Geometry check sheet. Reference: the model listing, model coordinates, mm. Face numbers are marked on the shaded views. A direction names the side the tool comes from. Give positions to 0.01 mm unless a question says otherwise; leave off trailing zeros. Write each loop counter-clockwise with the first axis right and the second up, starting at its lowest first coordinate (ties: lowest second). Pieces come first, ordered by that corner, then holes.
(1) Depth check by flat-ended pin: P1, Ø1.8, axis at x = 0, y = 6, coming from the -Z side; P2, Ø10, axis at x = 8, z = 18, coming from the +Y side; P3, Ø10, axis at x = 9.5, z = 1.5, coming from the +Y side; P4, Ø1.5, axis at x = 3, z = 2.5, coming from the +Y side. Enter the tip coordinate at first touch or a pass-through.
(2) Mould release check, pull along X, two halves, no side actions. Record for the marked faces 1, 2 and 3: +X half, -X half, draft (parallel to the pull), parting line (faces both ways), or undercut.
(3) Cross-section at A-A (y = 0). Record the boundary of the cut face in (x, z), and give its area (3 significant figures).
(4) Cross-section at D-D (x = -13). Record the boundary of the cut face in (y, z).
(5) Cross-section at C-C (x = -6.5). Record the boundary of the cut face in (y, z).
(6) Cross-section at B-B (x = 0). Record the boundary of the cut face in (y, z).
(7) Thickness scan on line 1 along Y through (x, z) = (0, 11); line 2 along Z through (x, y) = (3, 6); line 3 along X through (y, z) = (5, 3.5). Record the ranges inside material, lowest first.
(8) Tool access check on the marked faces 4, 5, 6, 7 and 8. Record the directions out of +Z, -Z, +X, -X, +Y, -Y that give a thin tool (end or side, any length) a straight path to the whole face; none if there is none.
```python
from build123d import *

# Parameters (mm, degrees)
SKIZZE1_R                       = 6
AUFSATZ_LINEAR_AUSTRAGEN1_DEPTH = 9
SKIZZE2_R                       = 3.925
AUFSATZ_LINEAR_AUSTRAGEN2_DEPTH = 7
SKIZZE3_R                       = 21
AUFSATZ_LINEAR_AUSTRAGEN3_DEPTH = 19
SKIZZE4_R                       = 15
SCHNITT_LINEAR_AUSTRAGEN2_DEPTH = 15.2
AUFSATZ_LINEAR_START            = -19
AUFSATZ_LINEAR_AUSTRAGEN4_DEPTH = 19
KREISMUSTER1_COUNT              = 9
SKETCH1_R                       = 1.5
CUT_EXTRUDE1_DEPTH              = 41.448579025
CUT_EXTRUDE2_START              = -3.8
SKETCH2_R                       = 2.25
CUT_EXTRUDE2_DEPTH              = 37.648579025
CUT_EXTRUDE3_START              = -3.8
CUT_EXTRUDE3_DEPTH              = 3.8


# Read off the part's stored shape, not the designer's step: Cut-Extrude3
with BuildPart() as part:
    # Skizze1 → Aufsatz-Linear austragen1 (new body)
    with BuildSketch(Plane.XY):
        Circle(SKIZZE1_R)
    extrude(amount=AUFSATZ_LINEAR_AUSTRAGEN1_DEPTH)

    # Skizze2 → Aufsatz-Linear austragen2 (add)
    with BuildSketch(Plane(origin=(0, 0, 0), x_dir=(-1, 0, 0), z_dir=(0, 0, -1))):
        Circle(SKIZZE2_R)
    extrude(amount=AUFSATZ_LINEAR_AUSTRAGEN2_DEPTH)

    # Skizze3 → Aufsatz-Linear austragen3 (add)
    with BuildSketch(Plane.XY.offset(9)):
        Circle(SKIZZE3_R)
    extrude(amount=AUFSATZ_LINEAR_AUSTRAGEN3_DEPTH)

    # Skizze4 → Schnitt-Linear austragen2 (cut)
    with BuildSketch(Plane.XY.offset(28)):
        Circle(SKIZZE4_R)
    extrude(amount=-SCHNITT_LINEAR_AUSTRAGEN2_DEPTH, mode=Mode.SUBTRACT)

    # Skizze6 → Aufsatz-Linear austragen4 (add)
    with BuildSketch(Plane.XY.offset(28).offset(AUFSATZ_LINEAR_START)):
        with BuildLine():
            Line((1.5, 25), (-1.5, 25))
            Line((-1.5, 25), (-1.5, 20.946360066))
            ThreePointArc((-1.5, 20.946360066), (0, 21), (1.5, 20.946360066))
            Line((1.5, 20.946360066), (1.5, 25))
        make_face()
    aufsatz_linear_austragen4 = extrude(amount=AUFSATZ_LINEAR_AUSTRAGEN4_DEPTH)

    # Kreismuster1: Aufsatz-Linear austragen4 ×9 about axis
    kreismuster1_axis = Axis((0, 0, 0), (0, 0, 1))
    for i in range(1, KREISMUSTER1_COUNT):
        add(aufsatz_linear_austragen4.rotate(kreismuster1_axis, i * 360 / KREISMUSTER1_COUNT))

    # Sketch1 → Cut-Extrude1 (cut, through all)
    with BuildSketch(Plane.XY.offset(12.8)):
        with Locations((-6, 0)):
            Circle(SKETCH1_R)
        with Locations((0, 6)):
            Circle(SKETCH1_R)
        with Locations((6, 0)):
            Circle(SKETCH1_R)
        with Locations((0, -6)):
            Circle(SKETCH1_R)
    extrude(amount=-CUT_EXTRUDE1_DEPTH, mode=Mode.SUBTRACT)

    # Sketch2 → Cut-Extrude2 (cut, through all)
    with BuildSketch(Plane.XY.offset(12.8).offset(CUT_EXTRUDE2_START)):
        with Locations((0, 6)):
            Circle(SKETCH2_R)
        with Locations((6, 0)):
            Circle(SKETCH2_R)
        with Locations((0, -6)):
            Circle(SKETCH2_R)
        with Locations((-6, 0)):
            Circle(SKETCH2_R)
    extrude(amount=-CUT_EXTRUDE2_DEPTH, mode=Mode.SUBTRACT)

    # Cut-Extrude3 outline → Cut-Extrude3 (cut)
    with BuildSketch(Plane(origin=(0, 0, 9), x_dir=(-1, 0, 0), z_dir=(0, 0, -1)).offset(CUT_EXTRUDE3_START)):
        with BuildLine():
            Line((7.72740661, 2.070552361), (14.488887394, 3.882285677))
            ThreePointArc((14.488887394, 3.882285677), (10.606601718, 10.606601718), (3.882285677, 14.488887394))
            Line((3.882285677, 14.488887394), (2.070552361, 7.72740661))
            ThreePointArc((2.070552361, 7.72740661), (5.656854249, 5.656854249), (7.72740661, 2.070552361))
        make_face()
        with BuildLine():
            ThreePointArc((3.882285677, -14.488887394), (10.606601718, -10.606601718), (14.488887394, -3.882285677))
            Line((14.488887394, -3.882285677), (7.72740661, -2.070552361))
            ThreePointArc((7.72740661, -2.070552361), (5.656854249, -5.656854249), (2.070552361, -7.72740661))
            Line((2.070552361, -7.72740661), (3.882285677, -14.488887394))
        make_face()
        with BuildLine():
            Line((-2.070552361, 7.72740661), (-3.882285677, 14.488887394))
            ThreePointArc((-3.882285677, 14.488887394), (-10.606601718, 10.606601718), (-14.488887394, 3.882285677))
            Line((-14.488887394, 3.882285677), (-7.72740661, 2.070552361))
            ThreePointArc((-7.72740661, 2.070552361), (-5.656854249, 5.656854249), (-2.070552361, 7.72740661))
        make_face()
        with BuildLine():
            ThreePointArc((-14.488887394, -3.882285677), (-10.606601718, -10.606601718), (-3.882285677, -14.488887394))
            Line((-3.882285677, -14.488887394), (-2.070552361, -7.72740661))
            ThreePointArc((-2.070552361, -7.72740661), (-5.656854249, -5.656854249), (-7.72740661, -2.070552361))
            Line((-7.72740661, -2.070552361), (-14.488887394, -3.882285677))
        make_face()
    extrude(amount=CUT_EXTRUDE3_DEPTH, mode=Mode.SUBTRACT)


solid = part.part
```
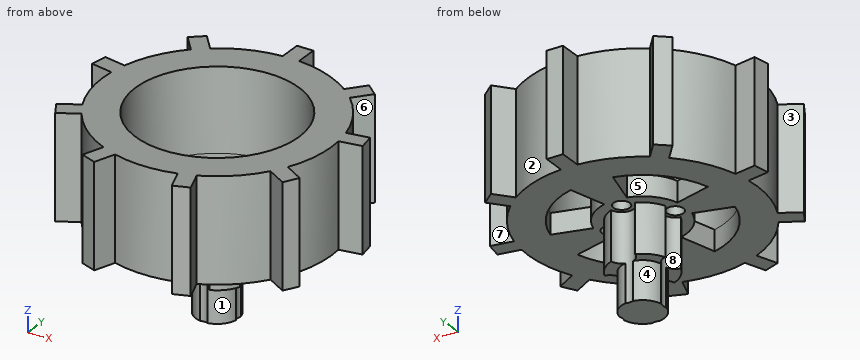
Reply:
1. P1: passes through
1. P2: stops at y = 20.78
1. P3: stops at y = 3.97
1. P4: stops at y = 5.56
2. face 1: +X half
2. face 2: undercut
2. face 3: -X half
3. outline: (-21, 9) - (-7.5, 9) - (-7.5, 12.8) - (-15, 12.8) - (-15, 28) - (-21, 28) - close; (-4.5, 9) - (-3.75, 9) - (-3.75, -7) - (3.75, -7) - (3.75, 9) - (4.5, 9) - (4.5, 12.8) - (-4.5, 12.8) - close; (7.5, 9) - (21, 9) - (21, 28) - (15, 28) - (15, 12.8) - (7.5, 12.8) - close
3. area: 439 mm2
4. outline: (-16.49, 9) - (-7.48, 9) - (-7.48, 28) - (-16.49, 28) - close; (-3.48, 9) - (3.48, 9) - (3.48, 12.8) - (-3.48, 12.8) - close; (7.48, 9) - (17.83, 9) - (17.83, 28) - (7.48, 28) - close
5. outline: (-22.24, 9) - (-13.52, 9) - (-13.52, 28) - (-22.24, 28) - close; (-4.66, 9) - (-1.41, 9) - (-1.41, 12.8) - (-4.66, 12.8) - close; (1.41, 9) - (4.66, 9) - (4.66, 12.8) - (1.41, 12.8) - close; (13.52, 9) - (19.97, 9) - (19.97, 28) - (13.52, 28) - close
6. outline: (-21, 9) - (-7.5, 9) - (-7.5, 12.8) - (-15, 12.8) - (-15, 28) - (-21, 28) - close; (-4.5, 9) - (-3.75, 9) - (-3.75, -7) - (3.75, -7) - (3.75, 9) - (4.5, 9) - (4.5, 12.8) - (-4.5, 12.8) - close; (7.5, 9) - (25, 9) - (25, 28) - (15, 28) - (15, 12.8) - (7.5, 12.8) - close
7. line 1: y = -21 to -7.5, -4.5 to 4.5, 7.5 to 25
7. line 2: z = 9 to 12.8
7. line 3: x = -3.32 to -2.02, 2.02 to 3.32
8. face 4: -Z, -X, +Y
8. face 5: +Z, -Z
8. face 6: +Z, -Z, +X
8. face 7: +Z, -Z, +Y
8. face 8: -Z, -X
